```python
from build123d import *

# Parameters (mm, degrees)
SKETCH_1_W          = 20
SKETCH_1_H          = 5
EXTRUDE_1_DEPTH     = 3
SKETCH_2_R          = 1.5
CUT_EXTRUDE_1_DEPTH = 3
CHAMFER_1_SIZE      = 1
CHAMFER_2_SIZE      = 1


with BuildPart() as part:
    # 草图1 → 凸台-拉伸1 (new body)
    with BuildSketch(Plane.XY):
        with Locations((-6.4536035, -0.430232558)):
            Rectangle(SKETCH_1_W, SKETCH_1_H)
    extrude(amount=EXTRUDE_1_DEPTH)

    # 草图2 → 切除-拉伸1 (cut)
    with BuildSketch(Plane.XY.offset(3)):
        with Locations((0.5463965, -0.430232558)):
            Circle(SKETCH_2_R)
    extrude(amount=-CUT_EXTRUDE_1_DEPTH, mode=Mode.SUBTRACT)

    # 倒角1
    chamfer_1_edges = [part.edges().sort_by_distance(p)[0] for p in [
        (3.5463965, -2.930232558, 1.5),
    ]]
    chamfer(chamfer_1_edges, length=CHAMFER_1_SIZE)

    # 倒角2
    chamfer_2_edges = [part.edges().sort_by_distance(p)[0] for p in [
        (3.5463965, 2.069767442, 1.5),
    ]]
    chamfer(chamfer_2_edges, length=CHAMFER_2_SIZE)


solid = part.part
```
CAD build for the part. Positions are in the model's coordinates, mm. Coordinates: 2 decimals unless noted, no trailing zeros. Loops run counter-clockwise (first coordinate to the right, second up) from the corner with the lowest first, then second, coordinate; pieces in that order, holes last. Notation, with made-up numbers: (73, 88.25) - (95, 88.25) arc R20 cw to (95, 107.25) - close; hole circle Ø5 at (15.25, 79). An arc over 180 degrees is marked (long way). Use CSV: the item, a comma, the result in double quotes. Start each with the question number.
Q1. Cut at C-C, the plane z = 2.25. List the corners of the cut face in (x, y).
Q2. Two-plate mould, pull along X, no slides. Class faces 1 (the flat face through (3.546, 0, 1)), 2 (the cylindrical face through (1.932, -1.005, 1.521)), 3 (the flat face through (-7, 2.07, 1)): +X half, -X half, draft (parallel to the pull), parting line (faces both ways), or undercut.
Q3. Cut at D-D, the plane y = 1.4. List the corners of the cut face in (x, z), then the cut area to 3 significant figures.
Q4. Cut at B-B, the plane x = 0. List the corners of the cut face in (y, z).
Q5. Probe probe 1 along X at (y, z) = (-0.35, 1.5); probe 2 along Y at (x, z) = (-0.5, 2.15); probe 3 along X at (y, z) = (-1.5, 0.7). List the from-to ranges inside material, lowest first. Write a range as from..to.
Q6. Cut at A-A, the plane y = -1.25. List the corners of the cut face in (x, z), then the cut area to 3 significant figures.
Here are the results:
1,outline,"(-16.45, -2.93) - (2.55, -2.93) - (3.55, -1.93) - (3.55, 1.07) - (2.55, 2.07) - (-16.45, 2.07) - close; hole circle Ø3 at (0.55, -0.43)"
2,face 1,"+X half"
2,face 2,"undercut"
2,face 3,"draft"
3,outline,"(-16.45, 0) - (3.22, 0) - (3.22, 3) - (-16.45, 3) - close"
3,area,"59.0 mm2"
4,outline,"(-2.93, 0) - (-1.83, 0) - (-1.83, 3) - (-2.93, 3) - close; (0.97, 0) - (2.07, 0) - (2.07, 3) - (0.97, 3) - close"
5,probe 1,"-16.45..-0.95, 2.04..3.55"
5,probe 2,"-2.93..-1.5, 0.64..2.07"
5,probe 3,"-16.45..-0.51, 1.6..3.55"
6,outline,"(-16.45, 0) - (-0.71, 0) - (-0.71, 3) - (-16.45, 3) - close; (1.8, 0) - (3.55, 0) - (3.55, 3) - (1.8, 3) - close"
6,area,"52.5 mm2"
